from build123d import *

# Parameters (mm, degrees)
ESQUISSE1_W             = 46.4
ESQUISSE1_H             = 52
EXTRUSION1_DEPTH        = 2
ESQUISSE2_R             = 2
ENL_V_MAT_EXTRU_1_DEPTH = 3
ENL_V_MAT_EXTRU_2_DEPTH = 3
CONG_1_R                = 2


with BuildPart() as part:
    # Esquisse1 → Extrusion1 (new body)
    with BuildSketch(Plane.XY):
        Rectangle(ESQUISSE1_W, ESQUISSE1_H)
    extrude(amount=EXTRUSION1_DEPTH)

    # Esquisse2 → Enlèv. mat.-Extru.1 (cut, through all)
    with BuildSketch(Plane.XY.offset(2)):
        with Locations((-20, 23)):
            Circle(ESQUISSE2_R)
        with Locations((20, 23)):
            Circle(ESQUISSE2_R)
    extrude(amount=-ENL_V_MAT_EXTRU_1_DEPTH, mode=Mode.SUBTRACT)

    # Esquisse3 → Enlèv. mat.-Extru.2 (cut, through all)
    with BuildSketch(Plane.XY.offset(2)):
        with BuildLine():
            Line((2, 23.5), (2, 22.5))
            ThreePointArc((2, 22.5), (0, 20.5), (-2, 22.5))
            Line((-2, 22.5), (-2, 23.5))
            ThreePointArc((-2, 23.5), (0, 25.5), (2, 23.5))
        make_face()
        with BuildLine():
            Line((2, -1.5), (2, -2.5))
            ThreePointArc((2, -2.5), (0, -4.5), (-2, -2.5))
            Line((-2, -2.5), (-2, -1.5))
            ThreePointArc((-2, -1.5), (0, 0.5), (2, -1.5))
        make_face()
    extrude(amount=-ENL_V_MAT_EXTRU_2_DEPTH, mode=Mode.SUBTRACT)

    # Congé1
    cong_1_edges = [part.edges().sort_by_distance(p)[0] for p in [
        (-23.2, 26, 1),
        (23.2, 26, 1),
        (23.2, -26, 1),
        (-23.2, -26, 1),
    ]]
    fillet(cong_1_edges, radius=CONG_1_R)


solid = part.part
Verification items for the finished model (mm, model axes). A direction names the side the tool comes from. Give positions to 0.01 mm unless a question says otherwise; leave off trailing zeros. Write each loop counter-clockwise with the first axis right and the second up, starting at its lowest first coordinate (ties: lowest second). Pieces come first, ordered by that corner, then holes. Notation, with made-up numbers: M 61.5,-23.5 L 96.5,-23.5 A15 cw 96.5,5.5 Z; hole C 45.5,76.25 d11. An arc over 180 degrees is marked long. Put each result on its own line as item: value. Start each with the question number.
1. Draft check along X on faces 1 (the face through (-22.63, -25.4, 1.01)), 2 (the face through (23.2, 0, 1)), 3 (the face through (0, 0.5, 1)). Enter one of: +X half, -X half, draft (parallel to the pull), parting line (faces both ways), or undercut.
2. Section check C-C (x = 20). Record the cut outline in (y, z), and give its area (3 significant figures).
3. Section check A-A (x = 0). Record the cut outline in (y, z), and give its area (3 significant figures).
4. Set-up check for faces 4 (the face through (0, -5, 0)), 5 (the face through (0, -4.5, 1)): record each of +Z, -Z, +X, -X, +Y, -Y from which the full face is reachable in a straight line by a thin tool's end or side.
5. Section check B-B (z = 1.5). Record the cut outline in (x, y), and give its area (3 significant figures).
6. Scan lines: line 1 along Y through (x, z) = (-20, 0.9); line 2 along Y through (x, z) = (19, 1.65); line 3 along X through (y, z) = (-3, 1.9). Record each from-to range of solid material in increasing order. Write a range as [from, to].
Answer list:
1. face 1: -X half
1. face 2: +X half
1. face 3: undercut
2. outline: M -26,0 L 21,0 L 21,2 L -26,2 Z; M 25,0 L 26,0 L 26,2 L 25,2 Z
2. area: 96.0 mm2
3. outline: M -26,0 L -4.5,0 L -4.5,2 L -26,2 Z; M 0.5,0 L 20.5,0 L 20.5,2 L 0.5,2 Z; M 25.5,0 L 26,0 L 26,2 L 25.5,2 Z
3. area: 84.0 mm2
4. face 4: -Z, +X, -X, +Y, -Y
4. face 5: +Z, -Z
5. outline: M -23.2,-24 A2 ccw -21.2,-26 L 21.2,-26 A2 ccw 23.2,-24 L 23.2,24 A2 ccw 21.2,26 L -21.2,26 A2 ccw -23.2,24 Z; hole C -20,23 d4; hole M -2,-2.5 A2 ccw 2,-2.5 L 2,-1.5 A2 ccw -2,-1.5 Z; hole M -2,22.5 A2 ccw 2,22.5 L 2,23.5 A2 ccw -2,23.5 Z; hole C 20,23 d4
5. area: 2,350 mm2
6. line 1: [-26, 21], [25, 26]
6. line 2: [-26, 21.27], [24.73, 26]
6. line 3: [-23.2, -1.94], [1.94, 23.2]
